For this review, use the dimensioned drawing (mm, ordinates from the lowest corner) and the shaded views. Coordinates: 2 decimals unless noted, no trailing zeros. Order: outer loops, then holes, each group sorted by start corner. A loop starts at its lowest first (then second) coordinate and runs counter-clockwise, first axis right, second up. Notation, with made-up numbers: (71, 71.5) -> (122, 71.5) arc R38 ccw to (122, 110.5) -> close; hole circle Ø4 at (41, 35). An arc over 180 degrees is marked (long way). Use one line per item in the form item = value. Start each with the question number.
(1) Take a section at B-B (x = 87). State the section outline as (y, z) points, then the cut area to 3 significant figures.
(2) Take a section at A-A (y = 2). State the section outline as (x, z) points, then the cut area to 3 significant figures.
(3) Wall thickness on line 1 along Z through (x, y) = (150, 1.4); line 2 along X through (y, z) = (2.4, 170.5); line 3 along Z through (x, y) = (85.5, 4.7): over which ranges is each line inside the solid? List them lowest first.
(4) Take a section at C-C (z = 185). State the section outline as (x, y) points.
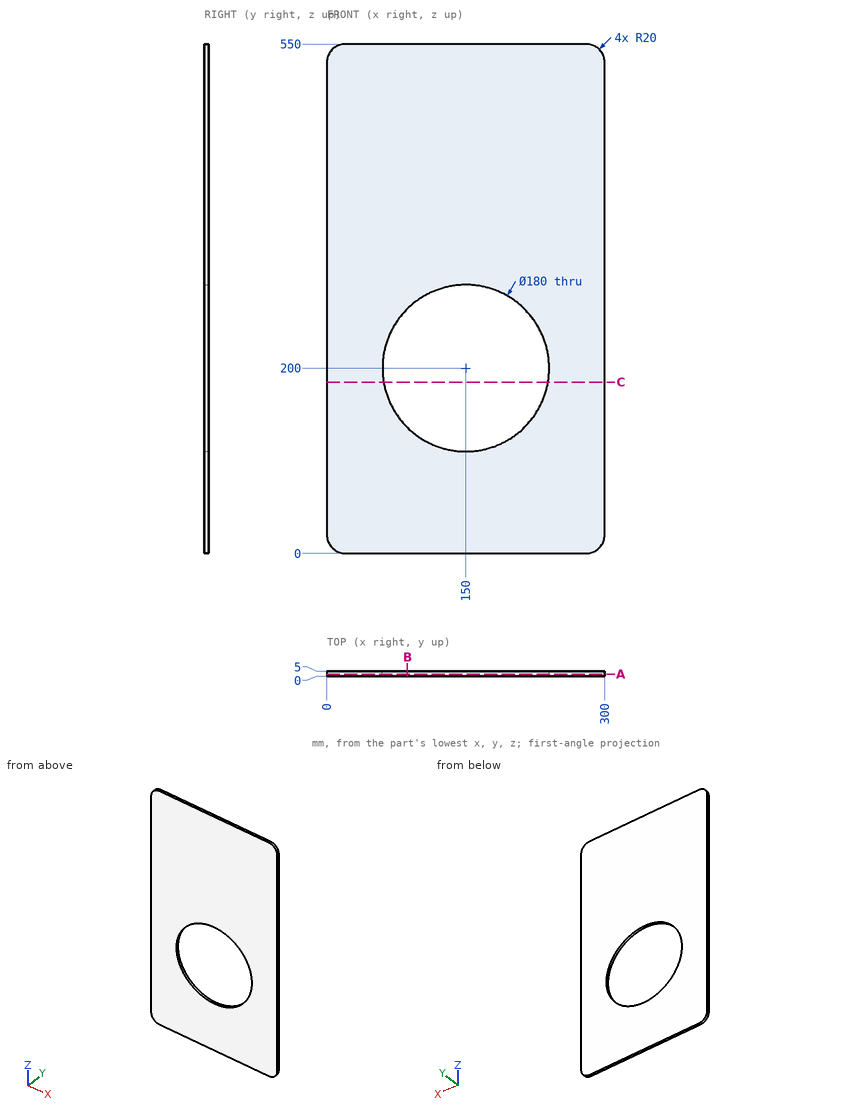
Findings:
q1.outline = (0, 0) -> (5, 0) -> (5, 135.73) -> (0, 135.73) -> close; (0, 264.27) -> (5, 264.27) -> (5, 550) -> (0, 550) -> close
q1.area = 2,110 mm²
q2.outline = (0, 20) arc R20 ccw to (20, 0) -> (280, 0) arc R20 ccw to (300, 20) -> (300, 530) arc R20 ccw to (280, 550) -> (20, 550) arc R20 ccw to (0, 530) -> close; hole circle Ø180 at (150, 200)
q2.area = 139,000 mm²
q3.line_1 = 0 to 110, 290 to 550
q3.line_2 = 0 to 64.97, 235.03 to 300
q3.line_3 = 0 to 137.23, 262.77 to 550
q4.outline = (0, 0) -> (61.26, 0) -> (61.26, 5) -> (0, 5) -> close; (238.74, 0) -> (300, 0) -> (300, 5) -> (238.74, 5) -> close
